Work out the finished part from the listing and answer in its coordinate system (mm). A direction names the side the tool comes from. Round coordinates to 2 decimals unless told otherwise and drop trailing zeros. Write each loop counter-clockwise with the first axis right and the second up, starting at its lowest first coordinate (ties: lowest second). Pieces come first, ordered by that corner, then holes.
1. Find section B-B (y = 0). Write down the section's boundary in (x, z).
2. A tool of negligible diameter and unlimited length cuts with its end or side. For faces 5 (the face through (1, 1.5, 1)), 6 (the face through (2, -2, 0)), from which of +Z, -Z, +X, -X, +Y, -Y can it reach the whole face along a straight path? Write none if from no direction.
3. A flat-ended cylindrical pin translates along its axis: pin 1 Ø1 at (y, z) = (3.5, 1) entering from -X. Find the tip coordinate at first contact, or state that the pin passes through.
4. Determine the mould class of faces 1 (the face through (7, 0, 2)), 2 (the face through (-3.5, 0, 1)), 3 (the face through (9.75, 0.05, 0.99)), 4 (the face through (15, 0, 1)) for opening direction X: pulls with the +X half, pulls with the -X half, needs draft (parallel to the pull), parting line crosses it, or undercut.
5. Find section D-D (x = 3.75). Write down the section's boundary in (y, z), and give its area (3 significant figures).
6. Find section C-C (z = 0.35). Write down the section's boundary in (x, y).
7. Straight lines are drawn through the part: probe 1 along Y at (x, z) = (3.25, 0.45); probe 2 along Y at (x, z) = (11, 1.2); probe 3 along X at (y, z) = (-0.25, 0.4). For each, find the intervals that lie inside material, in ascending order.
8. Find section A-A (x = 11). Write down the section's boundary in (y, z), and give its area (3 significant figures).
```python
from build123d import *

# Parameters (mm, degrees)
F0_R     = 1.25
F1_DEPTH = 2
F2_SIZE2 = 1.3397459622
F2_SIZE  = 5


with BuildPart() as f1:
    # F0 (on Top) → F1 (new body)
    with BuildSketch(Plane.XY):
        Polygon((15, -5), (15, 5), (-5, 5), (-10, 2.5), (-10, -2.5), (-5, -5), align=None)
        with BuildLine():
            ThreePointArc((-2, -1.5), (-3.5, 0), (-2, 1.5))
            Line((-2, 1.5), (5, 1.5))
            ThreePointArc((5, 1.5), (6.5, 0), (5, -1.5))
            Line((5, -1.5), (-2, -1.5))
        make_face(mode=Mode.SUBTRACT)
        with Locations((11, 0)):
            Circle(F0_R, mode=Mode.SUBTRACT)
    extrude(amount=F1_DEPTH)

    # F2
    f2_edges = [f1.edges().sort_by_distance(p)[0] for p in [
        (-10, 0, 2),
    ]]
    f2_side = f1.faces().sort_by_distance((14.730742, 0, 2))[0]
    chamfer(f2_edges, length=F2_SIZE, length2=F2_SIZE2, reference=f2_side)


solid = f1.part
```
Worked answers:
1. outline: (-10, 0) - (-3.5, 0) - (-3.5, 2) - (-5, 2) - (-10, 0.66) - close; (6.5, 0) - (9.75, 0) - (9.75, 2) - (6.5, 2) - close; (12.25, 0) - (15, 0) - (15, 2) - (12.25, 2) - close
2. face 5: +Z, -Z
2. face 6: -Z, +X, -X, +Y, -Y
3. pin 1: stops at x = -8.99
4. face 1: needs draft
4. face 2: undercut
4. face 3: undercut
4. face 4: pulls with the +X half
5. outline: (-5, 0) - (-1.5, 0) - (-1.5, 2) - (-5, 2) - close; (1.5, 0) - (5, 0) - (5, 2) - (1.5, 2) - close
5. area: 14.0 mm2
6. outline: (-10, -2.5) - (-5, -5) - (15, -5) - (15, 5) - (-5, 5) - (-10, 2.5) - close; hole (-2, -1.5) - (5, -1.5) arc R1.5 ccw to (5, 1.5) - (-2, 1.5) arc R1.5 ccw to start; hole circle Ø2.5 at (11, 0)
7. probe 1: y = -5 to -1.5, 1.5 to 5
7. probe 2: y = -5 to -1.25, 1.25 to 5
7. probe 3: x = -10 to -3.48, 6.48 to 9.78, 12.22 to 15
8. outline: (-5, 0) - (-1.25, 0) - (-1.25, 2) - (-5, 2) - close; (1.25, 0) - (5, 0) - (5, 2) - (1.25, 2) - close
8. area: 15.0 mm2
